Could you check a few things on this drawing? It's one solid part, dimensions in mm from its lowest x, y, z. A direction names the side the tool comes from. Coordinates: 2 decimals unless noted, no trailing zeros. Write each loop counter-clockwise with the first axis right and the second up, starting at its lowest first coordinate (ties: lowest second). Pieces come first, ordered by that corner, then holes. Notation, with made-up numbers: M 85,26 L 138,26 A23 ccw 138,39 Z; hole C 68,4 d7. An arc over 180 degrees is marked long. Use a Markdown table: item, result.
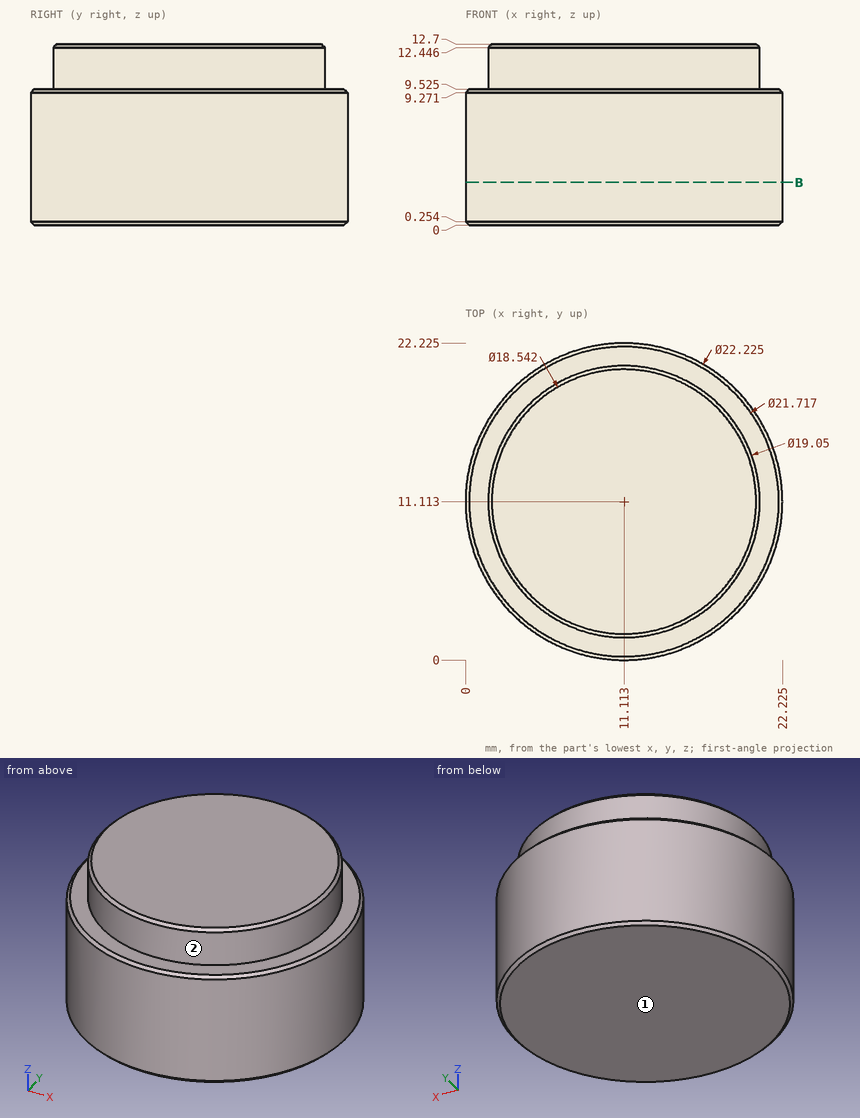
1. Which directions (+Z, -Z, +X, -X, +Y, -Y) give clear straight access to the entire face, cutting with the end or side of a thin tool? Please do the marked faces 1 and 2.
Answers follow:
| item | result |
|---|---|
| face 1 | -Z, +X, -X, +Y, -Y |
| face 2 | +Z |
2. Suppose I cut it at B-B on z = 3. Write out the boundary of the cut face in (x, y) (1 decimal).
Answers follow:
| item | result |
|---|---|
| outline | C 11.1,11.1 d22.2 |
3. Will these pins go through, and if not, where does the flat tip stop? pin 1 Ø5 at (y, z) = (9.5, 5.5) entering from -X; pin 2 Ø6 at (y, z) = (15.5, 4.5) entering from -X; pin 3 Ø3 at (y, z) = (18, 9) entering from +X; pin 4 Ø5 at (y, z) = (5.5, 3.5) entering from -X (1 decimal).
Answers follow:
| item | result |
|---|---|
| pin 1 | stops at x = 0 |
| pin 2 | stops at x = 0.09 |
| pin 3 | stops at x = 20.83 |
| pin 4 | stops at x = 0.4 |
4. I need wall thicknesses on probe 1 along Z at (x, y) = (1.5, 11.25) (1 decimal); probe 2 along Y at (x, z) = (3, 10.25) (1 decimal); probe 3 along Y at (x, z) = (15.25, 10.5) (1 decimal). Which ranges of each line are inside material? Lowest first, please.
Answers follow:
| item | result |
|---|---|
| probe 1 | z = 0 to 9.5 |
| probe 2 | y = 6.1 to 16.1 |
| probe 3 | y = 2.5 to 19.7 |
